Part model, mm, in its own coordinate system. Face numbers are marked on the shaded views. Round coordinates to 2 decimals unless told otherwise and drop trailing zeros. Write each loop counter-clockwise with the first axis right and the second up, starting at its lowest first coordinate (ties: lowest second). Pieces come first, ordered by that corner, then holes.
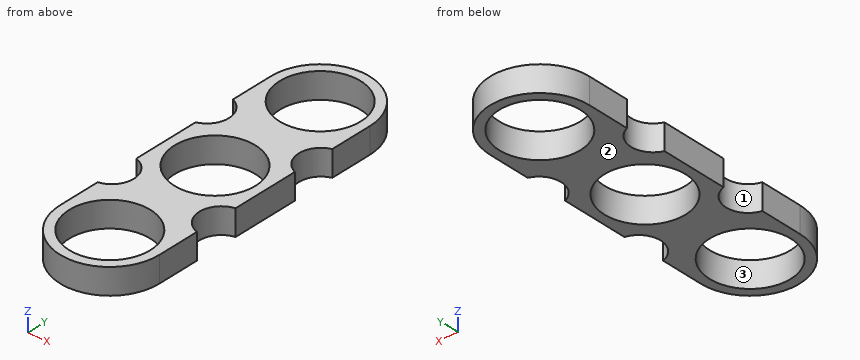
```python
from build123d import *

# Parameters (mm, degrees)
F0_R     = 11.05
F1_DEPTH = 7


with BuildPart() as f1:
    # F0 (on Top) → F1 (new body)
    with BuildSketch(Plane.XY):
        with BuildLine():
            Line((13.55, 20.420315), (13.55, 31.752493))
            ThreePointArc((13.55, 31.752493), (0, 45.302493), (-13.55, 31.752493))
            Line((-13.55, 31.752493), (-13.55, 20.420315))
            ThreePointArc((-13.55, 20.420315), (-9.564712, 14.768684), (-13.55, 9.117053))
            Line((-13.55, 9.117053), (-13.55, -8.768295))
            ThreePointArc((-13.55, -8.768295), (-8.954747, -14.601535), (-13.55, -20.434774))
            Line((-13.55, -20.434774), (-13.55, -31.752493))
            ThreePointArc((-13.55, -31.752493), (0, -45.302493), (13.55, -31.752493))
            Line((13.55, -31.752493), (13.55, -20.434774))
            ThreePointArc((13.55, -20.434774), (8.954747, -14.601535), (13.55, -8.768295))
            Line((13.55, -8.768295), (13.55, 9.117053))
            ThreePointArc((13.55, 9.117053), (9.564712, 14.768684), (13.55, 20.420315))
        make_face()
        with Locations((0, -31.752493)):
            Circle(F0_R, mode=Mode.SUBTRACT)
        Circle(F0_R, mode=Mode.SUBTRACT)
        with Locations((0, 31.752493)):
            Circle(F0_R, mode=Mode.SUBTRACT)
    extrude(amount=F1_DEPTH)


solid = f1.part
```
Q1. Cut at B-B on x = 0. Write the cut outline in (y, z), plus the area to 3 significant figures.
Values follow:
outline: (-45.3, 0) - (-42.8, 0) - (-42.8, 7) - (-45.3, 7) - close; (-20.7, 0) - (-11.05, 0) - (-11.05, 7) - (-20.7, 7) - close; (11.05, 0) - (20.7, 0) - (20.7, 7) - (11.05, 7) - close; (42.8, 0) - (45.3, 0) - (45.3, 7) - (42.8, 7) - close
area: 170 mm2
Q2. Cut at C-C on z = 2.75. Write the cut outline in (x, y).
Values follow:
outline: (-13.55, -31.75) arc R13.55 ccw to (13.55, -31.75) - (13.55, -20.43) arc R6 cw to (13.55, -8.77) - (13.55, 9.12) arc R6 cw to (13.55, 20.42) - (13.55, 31.75) arc R13.55 ccw to (-13.55, 31.75) - (-13.55, 20.42) arc R6 cw to (-13.55, 9.12) - (-13.55, -8.77) arc R6 cw to (-13.55, -20.43) - close; hole circle Ø22.1 at (0, -31.75); hole circle Ø22.1 at (0, 0); hole circle Ø22.1 at (0, 31.75)
Q3. Cut at D-D on x = 8. Write the cut outline in (y, z) (1 decimal).
Values follow:
outline: (-42.7, 0) - (-39.4, 0) - (-39.4, 7) - (-42.7, 7) - close; (-24.1, 0) - (-7.6, 0) - (-7.6, 7) - (-24.1, 7) - close; (7.6, 0) - (24.1, 0) - (24.1, 7) - (7.6, 7) - close; (39.4, 0) - (42.7, 0) - (42.7, 7) - (39.4, 7) - close
Q4. Drop a flat-ended pin along its axis: pin 1 (5 mm diameter, centred on x = -3.5, y = 7.5, fed in from +Z). Give the stop position or say it passes through.
Values follow:
pin 1: passes through
Q5. Wall check: L1, parallel to Y at x = 0, z = 2.25; L2, parallel to Y at x = -5.5, z = 4.25; L3, parallel to X at y = -25.5, z = 4.5. Give the ranges that are in metal, low to high.
Values follow:
L1: y = -45.3 to -42.8, -20.7 to -11.05, 11.05 to 20.7, 42.8 to 45.3
L2: y = -44.14 to -41.34, -22.17 to -9.58, 9.58 to 22.17, 41.34 to 44.14
L3: x = -13.55 to -9.11, 9.11 to 13.55
Q6. Mould opens along X. For the marked faces 1, 2 and 3 say: +X half, -X half, draft (parallel to the pull), parting line (faces both ways), or undercut.
Values follow:
face 1: -X half
face 2: draft
face 3: undercut
Q7. Cut at A-A on y = 0. Write the cut outline in (x, z).
Values follow:
outline: (-13.55, 0) - (-11.05, 0) - (-11.05, 7) - (-13.55, 7) - close; (11.05, 0) - (13.55, 0) - (13.55, 7) - (11.05, 7) - close
